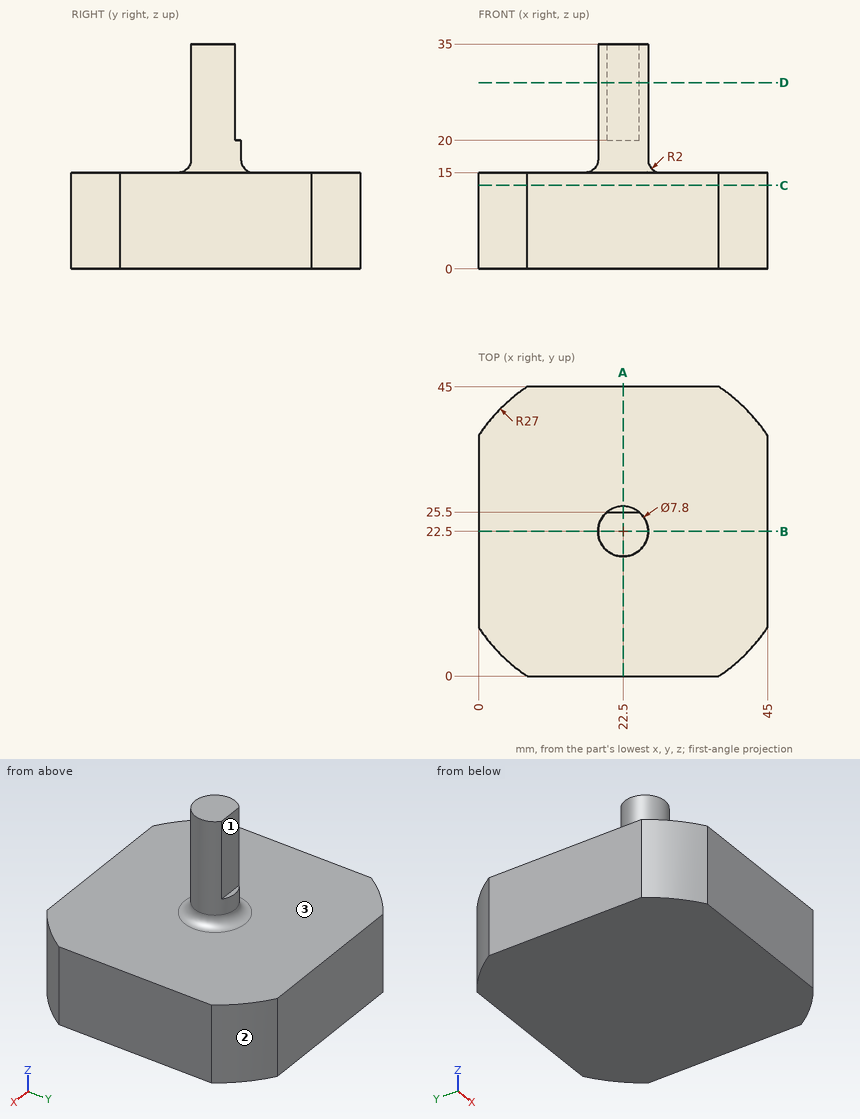
Verification items for this drawing (mm, ordinates from the low corner). A direction names the side the tool comes from. Coordinates: 2 decimals unless noted, no trailing zeros. Write each loop counter-clockwise with the first axis right and the second up, starting at its lowest first coordinate (ties: lowest second). Pieces come first, ordered by that corner, then holes. Notation, with made-up numbers: M 21,26.5 L 70,26.5 A19 cw 70,46.5 Z; hole C -30.5,-33 d8. An arc over 180 degrees is marked long. Use CSV: the item, a comma, the result in double quotes.
Q1. Set-up check for the marked faces 1, 2 and 3: record each of +Z, -Z, +X, -X, +Y, -Y from which the full face is reachable in a straight line by a thin tool's end or side.
Computed values:
face 1,"+Z, +X, -X, +Y"
face 2,"+Z, -Z, +X, +Y"
face 3,"+Z"
Q2. Section check C-C, the plane z = 13. Enter the section's corners in (x, y).
Computed values:
outline,"M 0,7.58 A27 ccw 7.58,0 L 37.42,0 A27 ccw 45,7.58 L 45,37.42 A27 ccw 37.42,45 L 7.58,45 A27 ccw 0,37.42 Z"
Q3. Section check D-D, the plane z = 29. Enter the section's corners in (x, y).
Computed values:
outline,"M 20.01,25.5 A3.9 ccw long 24.99,25.5 Z"
Q4. Section check B-B, the plane y = 22.5. Enter the section's corners in (x, z).
Computed values:
outline,"M 0,0 L 45,0 L 45,15 L 28.4,15 A2 cw 26.4,17 L 26.4,35 L 18.6,35 L 18.6,17 A2 cw 16.6,15 L 0,15 Z"
Q5. Thickness scan on line 1 along Z through (x, y) = (6.5, 21); line 2 along Y through (x, z) = (22, 24); line 3 along Y through (x, z) = (20, 28.5). Record the ranges inside material, lowest first. Write a range as [from, to].
Computed values:
line 1,"[0, 15]"
line 2,"[18.63, 25.5]"
line 3,"[19.51, 25.49]"
Q6. Go/stop test with flat-tipped pins: P1, Ø3, axis at x = 29.5, z = 18.5, coming from the +Y side; P2, Ø0.5, axis at x = 22.5, y = 26, coming from the +Z side; P3, Ø5, axis at y = 21, z = 23, coming from the -X side; P4, Ø4, axis at x = 23, z = 26, coming from the +Y side. Record where each tip stops, or that it passes through.
Computed values:
P1,"through"
P2,"z = 20"
P3,"x = 18.6"
P4,"y = 25.5"
Q7. Section check A-A, the plane x = 22.5. Enter the section's corners in (y, z), and give its area (3 significant figures).
Computed values:
outline,"M 0,0 L 45,0 L 45,15 L 28.4,15 A2 cw 26.4,17 L 26.4,20 L 25.5,20 L 25.5,35 L 18.6,35 L 18.6,17 A2 cw 16.6,15 L 0,15 Z"
area,"819 mm²"
